Here's how the part is built. I have some questions about the finished solid (model axes, mm). A direction names the side the tool comes from. Coordinates: 2 decimals unless noted, no trailing zeros. Write each loop counter-clockwise with the first axis right and the second up, starting at its lowest first coordinate (ties: lowest second). Pieces come first, ordered by that corner, then holes. Notation, with made-up numbers: (-23.5, 55) -> (29.5, 55) arc R13 cw to (29.5, 79) -> close; hole circle Ø1 at (-19.5, -22.5). An arc over 180 degrees is marked (long way). Answer in a Markdown table with one row per item. Add a question column.
from build123d import *

# Parameters (mm, degrees)
F0_W     = 150
F0_H     = 150
F1_DEPTH = 80
F2_T     = -5
F3_R     = 7.863992
F3_R_2   = 11.429543
F4_DEPTH = 25


with BuildPart() as f1:
    # F0 (on Top) → F1 (new body)
    with BuildSketch(Plane.XY):
        Rectangle(F0_W, F0_H)
    extrude(amount=F1_DEPTH)

    # F2
    f2_openings = [f1.faces().sort_by_distance(p)[0] for p in [
        (0, 0, 80),
    ]]
    offset(amount=F2_T, openings=f2_openings)

    # F3 (on face) → F4 (cut)
    with BuildSketch(Plane.XZ.offset(75)):
        with Locations((-27.252719, 56.159835)):
            Circle(F3_R)
        with Locations((9.724549, 53.455554)):
            Circle(F3_R_2)
    extrude(amount=-F4_DEPTH, mode=Mode.SUBTRACT)


solid = f1.part
Q1. Imagine slicing it at C-C on y = -61. Please give me the cut outline in (x, z).
Q2. I need wall thicknesses on line 1 (Y direction, x = -7, z = 7.5); line 2 (Z direction, x = 8.5, y = 47). Which ranges of each line are inside material? Lowest first, please. Write a range as [from, to].
Q3. Imagine slicing it at B-B on x = -26.5. Please give me the cut outline in (y, z).
Q4. If we mould it in two halves opening along X, with no side actions, what happens to faces 4 (the flat face through (70, -1, 42)), 5 (the flat face through (-1, -75, 39)), 6 (the flat face through (75, -1, 39))? For each: pulls with the +X half, pulls with the -X half, needs draft (parallel to the pull), parting line crosses it, or undercut.
Q5. I'm going to push flat-ended pins straight in: P1, Ø10, axis at x = -35, y = -24.5, coming from the +Z side; P2, Ø22.5, axis at x = 7, z = 45, coming from the -Y side; P3, Ø18.5, axis at x = 9.72, z = 53.46, coming from the -Y side. Where does each tip first touch, or does it pass through?
Q6. For faces 1 (the cylindrical face through (8.24, -72.54, 64.79)), 2 (the flat face through (-1, 1, 0)), 3 (the flat face through (-1, -70, 42)), which set-ups out of +Z, -Z, +X, -X, +Y, -Y let a thin tool reach every point of the face, with its end or its side?
Q7. Imagine slicing it at A-A on z = 22.5. Please give me the cut outline in (x, y), plus the area to 3 significant figures.
Result sheet:
| question | item | result |
|---|---|---|
| 1 | outline | (-75, 0) -> (75, 0) -> (75, 80) -> (70, 80) -> (70, 5) -> (-70, 5) -> (-70, 80) -> (-75, 80) -> close |
| 2 | line 1 | y = [-75, -70], [70, 75] |
| 2 | line 2 | z = [0, 5] |
| 3 | outline | (-75, 0) -> (75, 0) -> (75, 80) -> (70, 80) -> (70, 5) -> (-70, 5) -> (-70, 48.33) -> (-75, 48.33) -> close; (-75, 63.99) -> (-70, 63.99) -> (-70, 80) -> (-75, 80) -> close |
| 4 | face 4 | undercut |
| 4 | face 5 | needs draft |
| 4 | face 6 | pulls with the +X half |
| 5 | P1 | stops at z = 5 |
| 5 | P2 | stops at y = -75 |
| 5 | P3 | stops at y = 70 |
| 6 | face 1 | -Y |
| 6 | face 2 | -Z, +X, -X, +Y, -Y |
| 6 | face 3 | +Z |
| 7 | outline | (-75, -75) -> (75, -75) -> (75, 75) -> (-75, 75) -> close; hole (-70, -70) -> (70, -70) -> (70, 70) -> (-70, 70) -> close |
| 7 | area | 2,900 mm^2 |
